from build123d import *

# Parameters (mm, degrees)
F1_DEPTH    = 38.1
F2_T1_DEPTH = 38.1
F2_T3_DEPTH = 50.8
F3_T1_DEPTH = 38.1
F4_R        = 1.26999


# Not quite as in the source:
# - a fillet or chamfer that OpenCascade refuses, or shapes differently, is made with other operations: its cross-section is extruded or revolved along the edge and cut away or added
# - a fillet or chamfer is up to 0.001 mm smaller than in the source, because OpenCascade refuses the exact size


with BuildPart() as f1:
    # F0 (on Top) → F1 (new body)
    with BuildSketch(Plane.XY):
        Polygon((-37.2364, 25.4), (-37.2364, 0), (37.2364, 0), (37.2364, 12.7), (33.4264, 13.3497271487), (33.4264, 2.54), (30.226, 2.54), (30.226, 13.8954979536), (27.686, 14.3286493861), (27.686, 2.54), (23.9776, 2.54), (23.9776, 14.9610504775), (21.4376, 15.39420191), (21.4376, 2.54), (17.0942, 2.54), (17.0942, 16.1348908595), (14.5542, 16.568042292), (14.5542, 2.54), (9.8044, 2.54), (9.8044, 17.3780354707), (7.2644, 17.8111869031), (7.2644, 2.54), (1.7272, 2.54), (1.7272, 18.7554570259), (-0.8128, 19.1886084584), (-0.8128, 2.54), (-6.7564, 2.54), (-6.7564, 20.2021828104), (-9.2964, 20.6353342428), (-9.2964, 2.54), (-15.6464, 2.54), (-15.6464, 21.718212824), (-18.1864, 22.1513642565), (-18.1864, 2.54), (-24.5364, 2.54), (-24.5364, 23.2342428377), (-27.0764, 23.6673942701), (-27.0764, 2.54), (-33.4264, 2.54), (-33.4264, 24.9766666667), align=None)
    extrude(amount=F1_DEPTH)

    # F2: fillet of radius 2.54 on 14 edges, made by hand

    # F2_s2 → F2_t1 (join)
    with BuildSketch(Plane.XY):
        with BuildLine():
            ThreePointArc((-30.8864, 2.54), (-32.6824512242, 3.2839487758), (-33.4264, 5.08))
            Line((-33.4264, 5.08), (-33.4264, 2.54))
            Line((-33.4264, 2.54), (-30.8864, 2.54))
        make_face()
        with BuildLine():
            ThreePointArc((-27.0764, 5.08), (-27.8203487758, 3.2839487758), (-29.6164, 2.54))
            Line((-29.6164, 2.54), (-27.0764, 2.54))
            Line((-27.0764, 2.54), (-27.0764, 5.08))
        make_face()
        with BuildLine():
            ThreePointArc((-21.9964, 2.54), (-23.7924512242, 3.2839487758), (-24.5364, 5.08))
            Line((-24.5364, 5.08), (-24.5364, 2.54))
            Line((-24.5364, 2.54), (-21.9964, 2.54))
        make_face()
        with BuildLine():
            ThreePointArc((-18.1864, 5.08), (-18.9303487758, 3.2839487758), (-20.7264, 2.54))
            Line((-20.7264, 2.54), (-18.1864, 2.54))
            Line((-18.1864, 2.54), (-18.1864, 5.08))
        make_face()
        with BuildLine():
            ThreePointArc((-13.1064, 2.54), (-14.9024512242, 3.2839487758), (-15.6464, 5.08))
            Line((-15.6464, 5.08), (-15.6464, 2.54))
            Line((-15.6464, 2.54), (-13.1064, 2.54))
        make_face()
        with BuildLine():
            ThreePointArc((-9.2964, 5.08), (-10.0403487758, 3.2839487758), (-11.8364, 2.54))
            Line((-11.8364, 2.54), (-9.2964, 2.54))
            Line((-9.2964, 2.54), (-9.2964, 5.08))
        make_face()
        with BuildLine():
            ThreePointArc((-4.2164, 2.54), (-6.0124512242, 3.2839487758), (-6.7564, 5.08))
            Line((-6.7564, 5.08), (-6.7564, 2.54))
            Line((-6.7564, 2.54), (-4.2164, 2.54))
        make_face()
        with BuildLine():
            ThreePointArc((-0.8128, 5.08), (-1.5567487758, 3.2839487758), (-3.3528, 2.54))
            Line((-3.3528, 2.54), (-0.8128, 2.54))
            Line((-0.8128, 2.54), (-0.8128, 5.08))
        make_face()
        with BuildLine():
            ThreePointArc((4.2672, 2.54), (2.4711487758, 3.2839487758), (1.7272, 5.08))
            Line((1.7272, 5.08), (1.7272, 2.54))
            Line((1.7272, 2.54), (4.2672, 2.54))
        make_face()
        with BuildLine():
            ThreePointArc((7.2644, 5.08), (6.5204512242, 3.2839487758), (4.7244, 2.54))
            Line((4.7244, 2.54), (7.2644, 2.54))
            Line((7.2644, 2.54), (7.2644, 5.08))
        make_face()
        with BuildLine():
            ThreePointArc((12.3444, 2.54), (10.5483487758, 3.2839487758), (9.8044, 5.08))
            Line((9.8044, 5.08), (9.8044, 2.54))
            Line((9.8044, 2.54), (12.3444, 2.54))
        make_face()
        with BuildLine():
            ThreePointArc((14.5542, 5.08), (13.8102512242, 3.2839487758), (12.0142, 2.54))
            Line((12.0142, 2.54), (14.5542, 2.54))
            Line((14.5542, 2.54), (14.5542, 5.08))
        make_face()
    extrude(amount=F2_T1_DEPTH)

    # F2_s4 → F2_t3 (cut)
    with BuildSketch(Plane.XY.offset(-6.35)):
        with BuildLine():
            ThreePointArc((-37.2364, 2.54), (-36.4924512242, 0.7439487758), (-34.6964, 0))
            Line((-34.6964, 0), (-37.2364, 0))
            Line((-37.2364, 0), (-37.2364, 2.54))
        make_face()
        with BuildLine():
            ThreePointArc((34.6964, 0), (36.4924512242, 0.7439487758), (37.2364, 2.54))
            Line((37.2364, 2.54), (37.2364, 0))
            Line((37.2364, 0), (34.6964, 0))
        make_face()
    extrude(amount=F2_T3_DEPTH, mode=Mode.SUBTRACT)

    # F3: fillet of radius 1.778 on 6 edges, made by hand

    # F3_s2 → F3_t1 (join)
    with BuildSketch(Plane.XY):
        with BuildLine():
            ThreePointArc((17.0942, 4.318), (17.6149641431, 3.0607641431), (18.8722, 2.54))
            Line((18.8722, 2.54), (17.0942, 2.54))
            Line((17.0942, 2.54), (17.0942, 4.318))
        make_face()
        with BuildLine():
            ThreePointArc((19.6596, 2.54), (20.9168358569, 3.0607641431), (21.4376, 4.318))
            Line((21.4376, 4.318), (21.4376, 2.54))
            Line((21.4376, 2.54), (19.6596, 2.54))
        make_face()
        with BuildLine():
            ThreePointArc((23.9776, 4.318), (24.4983641431, 3.0607641431), (25.7556, 2.54))
            Line((25.7556, 2.54), (23.9776, 2.54))
            Line((23.9776, 2.54), (23.9776, 4.318))
        make_face()
        with BuildLine():
            ThreePointArc((25.908, 2.54), (27.1652358569, 3.0607641431), (27.686, 4.318))
            Line((27.686, 4.318), (27.686, 2.54))
            Line((27.686, 2.54), (25.908, 2.54))
        make_face()
        with BuildLine():
            ThreePointArc((30.226, 4.318), (30.7467641431, 3.0607641431), (32.004, 2.54))
            Line((32.004, 2.54), (30.226, 2.54))
            Line((30.226, 2.54), (30.226, 4.318))
        make_face()
        with BuildLine():
            ThreePointArc((31.6484, 2.54), (32.9056358569, 3.0607641431), (33.4264, 4.318))
            Line((33.4264, 4.318), (33.4264, 2.54))
            Line((33.4264, 2.54), (31.6484, 2.54))
        make_face()
    extrude(amount=F3_T1_DEPTH)

    # F4 (radius 1.27 in the source; OpenCascade refuses exactly that, so slightly less here)
    f4_edges = [f1.edges().sort_by_distance(p)[0] for p in [
        (33.4264, 13.349727, 19.05),
        (30.226, 13.895498, 19.05),
        (27.686, 14.328649, 19.05),
        (23.9776, 14.96105, 19.05),
        (21.4376, 15.394202, 19.05),
        (17.0942, 16.134891, 19.05),
        (14.5542, 16.568042, 19.05),
        (9.8044, 17.378035, 19.05),
        (7.2644, 17.811187, 19.05),
        (1.7272, 18.755457, 19.05),
        (-0.8128, 19.188608, 19.05),
        (-6.7564, 20.202183, 19.05),
        (-15.6464, 21.718213, 19.05),
        (-24.5364, 23.234243, 19.05),
        (-27.0764, 23.667394, 19.05),
        (-33.4264, 24.976667, 19.05),
        (-37.2364, 25.4, 19.05),
        (37.2364, 12.7, 19.05),
        (-9.2964, 20.635334, 19.05),
        (-18.1864, 22.151364, 19.05),
    ]]
    fillet(f4_edges, radius=F4_R)


solid = f1.part
For this review, take the finished solid that the model builds, in its own axes (mm). Give positions to 0.01 mm unless a question says otherwise; leave off trailing zeros. Loops run counter-clockwise (first coordinate to the right, second up) from the corner with the lowest first, then second, coordinate; pieces in that order, holes last. Notation, with made-up numbers: (8.5, -17) -> (25.5, -17) arc R9 ccw to (25.5, -2) -> close; hole circle Ø4 at (-24.5, 51.25). An arc over 180 degrees is marked (long way). One line per question, with ' | ' between items.
1) Insertion check: pin 1 Ø5.5 at (y, z) = (16, 9.5) entering from +X; pin 2 Ø1 at (x, z) = (-12.5, 26) entering from +Y; pin 3 Ø0.9 at (x, z) = (-4, 27) entering from +Y. Each pin has a flat end and moves straight along its axis. Give the tip position at first contact, or say it passes through.
Resolved:
pin 1: stops at x = 30.15 | pin 2: stops at y = 2.54 | pin 3: stops at y = 2.55
2) We need section C-C (x = -11). Write out the cut boundary in (y, z), plus the area to 3 significant figures.
Resolved:
outline: (0, 0) -> (2.68, 0) -> (2.68, 38.1) -> (0, 38.1) -> close | area: 102 mm2
3) The part is to be moulded in two halves that separate along X. For faces 1 (the flat face through (1, 10, 38.1)), 2 (the flat face through (-6.756, 12, 19)), say which applies: +X half, -X half, draft (parallel to the pull), parting line (faces both ways), or undercut.
Resolved:
face 1: draft | face 2: undercut
4) To check wall thickness, follow probe 1 along X at (y, z) = (19, 17); probe 2 along X at (y, z) = (18, 3); probe 3 along Y at (x, z) = (15.5, 30). State the ranges of each line that lie inside material, in increasing order.
Resolved:
probe 1: x = -37.24 to -33.43, -27.08 to -24.54, -18.19 to -15.65, -9.3 to -6.76 | probe 2: x = -37.24 to -33.43, -27.08 to -24.54, -18.19 to -15.65, -9.3 to -6.76, -0.77 to 1.69 | probe 3: y = 0 to 16.29
5) We need section B-B (x = -28.5). Write out the cut boundary in (y, z).
Resolved:
outline: (0, 0) -> (2.8, 0) -> (2.8, 38.1) -> (0, 38.1) -> close
6) We need section A-A (y = 6). Give the number of separate pieces and of enclosed holes in the cut face, plus the area to 3 significant figures.
Resolved:
separate pieces: 10 | enclosed holes: 0 | area: 1,060 mm2
